Autodesk Fusion 360 part; units mm, degrees
sketch "Sketch1" plane through (0, 0, 0) normal (0, 1, 0) x (1, 0, 0)
  line L0 (-20, -450) -> (-20, 0)
  arc A0 (20, 0) -> (-20, 0) centre (0, 0) ccw
  line L1 (20, 0) -> (20, -450)
  line L2 (20, -450) -> (-20, -450)
  point P0 (0, -200)
  point P1 (-15, -245)
  dimension "d1" = 20
  dimension "d2" = 450
  dimension "d3" = 200
  dimension "d9" = 45
  dimension "d10" = 15
extrude "Extrude1" add sketch "Sketch1" along normal blind 15
hole "Hole1" at (0, 0, 200) at (0, 0, 0) direction (0, 1, 0) diameter 15.526 depth 200 tip angle 118
hole "Hole2" at (-15, 0, 245) direction (0, 1, 0) diameter 7 depth 200 tip angle 118
pattern_linear "R-Pattern1" count 11 spacing 25 along (0, 0, 1) count 2 spacing 25 along (1, 0, 0) of "Hole2"
chamfer "Chamfer1" distance 2 angle 45 2 edges at (20, 7.5, 450) (-20, 7.5, 450)
Read the model definition and answer for the solid it produces. Units are mm, in the model's axes. Round coordinates to 2 decimals unless told otherwise and drop trailing zeros. Write each loop counter-clockwise with the first axis right and the second up, starting at its lowest first coordinate (ties: lowest second). Pieces come first, ordered by that corner, then holes.
1. The part is cut by section B-B, the plane y = 11.75. State how many separate pieces and enclosed holes the cut face has, then the cut area to 3 significant figures.
2. Determine the mould class of faces 1 (the face through (7.58, 7.6, 1.68)), 2 (the face through (0, 15, 212)), 3 (the face through (0, 7, -20)) for opening direction Z: pulls with the +Z half, pulls with the -Z half, needs draft (parallel to the pull), parting line crosses it, or undercut.
3. Straight lines are drawn through the part: L1, parallel to X at y = 3.5, z = 420; L2, parallel to Z at x = 0, y = 5.5; L3, parallel to Z at x = 16, y = 8.25. For each, find the intervals that lie inside material, in ascending order.
4. Given pin 1 Ø5 at (x, y) = (-0.5, 7.5) entering from -Z; pin 2 Ø8 at (x, y) = (14, 6) entering from -Z, each flat-ended and moving along its own axis, determine where each tip first touches the part or whether it passes through.
5. The part is cut by section A-A, the plane z = 200. Determine the outline of the cut face in (x, y).
Values:
1. separate pieces: 1
1. enclosed holes: 20
1. area: 17,600 mm2
2. face 1: undercut
2. face 2: needs draft
2. face 3: pulls with the -Z half
3. L1: x = -20 to -18.5, -11.5 to 6.5, 13.5 to 20
3. L2: z = -20 to -7.76, 7.76 to 192.24, 207.76 to 450
3. L3: z = -12 to 450
4. pin 1: stops at z = -20
4. pin 2: stops at z = -17.32
5. outline: (-20, 0) - (-7.76, 0) - (-7.76, 15) - (-20, 15) - close; (7.76, 0) - (20, 0) - (20, 15) - (7.76, 15) - close
